Design review of the part built by this model. Coordinates are the model's own, in mm. A direction names the side the tool comes from. Round coordinates to 2 decimals unless told otherwise and drop trailing zeros. Order: outer loops, then holes, each group sorted by start corner. A loop starts at its lowest first (then second) coordinate and runs counter-clockwise, first axis right, second up. Notation, with made-up numbers: M 34,9 L 90,9 A22 ccw 90,45 Z; hole C 36,-20 d3. An arc over 180 degrees is marked long. Use a Markdown table: item, result. Add a question column.
(1) The part is to be moulded in two halves that separate along X. For faces 4 (the face through (-46, 5, 0)), 5 (the face through (-44.8, 2, 20)), 6 (the face through (21.04, 1.04, 16.09)), 7 (the face through (-26.863, 1.035, 35.391)), say which applies: released by +X, released by -X, zero draft, split by the parting line, or undercut.
(2) Take a section at A-A (x = 0). Write out the cut boundary in (y, z), then the cut area to 3 significant figures.
(3) Take a section at B-B (z = 0). Write out the cut boundary in (x, y), then the cut area to 3 significant figures.
(4) Take a section at D-D (x = -18). Write out the cut boundary in (y, z), then the cut area to 3 significant figures.
(5) To check wall thickness, follow probe 1 along Z at (x, y) = (0, 1.75); probe 2 along X at (y, z) = (1.3, -23). State the ranges of each line that lie inside material, in increasing order. Write a range as from..to.
(6) For pin 1 (1.5 mm diameter, centred on x = 19, z = 45.5, fed in from -Y); pin 2 (1.5 mm diameter, centred on x = 47, y = 3.5, fed in from +Z); pin 3 (1.1 mm diameter, centred on y = 2.5, z = -21.5, fed in from -X); pin 4 (2.5 mm diameter, centred on y = 2.5, z = -46.5, fed in from +X), all flat-tipped, find the tip position at first contact; note any pin that passes through.
(7) Machinability: for faces 1 (the face through (46, 1.2, 20)), 2 (the face through (10, 2.1, -10)), 3 (the face through (9.8, 1, -4.1)), which of the approach directions +Z, -Z, +X, -X, +Y, -Y give a long, thin tool a straight path to every point of the face, cutting with its end or side? Answer none if there is none.
(8) Take a section at C-C (z = -33). Write out the cut boundary in (x, y).
```python
from build123d import *

# Parameters (mm, degrees)
SKETCH1_R           = 5
BOSS_EXTRUDE1_DEPTH = 2.1
BOSS_EXTRUDE2_DEPTH = 2.9
SKETCH3_W           = 10.2
SKETCH3_H           = 3.8
CUT_EXTRUDE1_DEPTH  = 3
CIRPATTERN1_COUNT   = 4
CHAMFER1_SIZE       = 1


with BuildPart() as part:
    # Sketch1 → Boss-Extrude1 (new body)
    with BuildSketch(Plane(origin=(0, 0, 0), x_dir=(1, 0, 0), z_dir=(0, 1, 0))):
        Polygon((-47.8, -41.4), (-47.8, 41.4), (-41.4, 41.4), (-41.4, 47.8), (41.4, 47.8), (41.4, 41.4), (47.8, 41.4), (47.8, -41.4), (41.4, -41.4), (41.4, -47.8), (-41.4, -47.8), (-41.4, -41.4), align=None)
        Circle(SKETCH1_R, mode=Mode.SUBTRACT)
        with BuildLine():
            Line((-30.971572875, -26.021825407), (-10.834000483, -5.884253014))
            ThreePointArc((-10.834000483, -5.884253014), (-9.821178524, -4.171534398), (-9.758876863, -2.182732778))
            ThreePointArc((-9.758876863, -2.182732778), (-10, 0), (-9.758876863, 2.182732778))
            ThreePointArc((-9.758876863, 2.182732778), (-9.821178524, 4.171534398), (-10.834000483, 5.884253014))
            Line((-10.834000483, 5.884253014), (-30.971572875, 26.021825407))
            ThreePointArc((-30.971572875, 26.021825407), (-35.330733729, 26.888916412), (-37.8, 23.193398282))
            Line((-37.8, 23.193398282), (-37.8, -23.193398282))
            ThreePointArc((-37.8, -23.193398282), (-35.330733729, -26.888916412), (-30.971572875, -26.021825407))
        make_face(mode=Mode.SUBTRACT)
        with BuildLine():
            Line((-26.021825407, -30.971572875), (-5.884253014, -10.834000483))
            ThreePointArc((-5.884253014, -10.834000483), (-4.171534398, -9.821178524), (-2.182732778, -9.758876863))
            ThreePointArc((-2.182732778, -9.758876863), (0, -10), (2.182732778, -9.758876863))
            ThreePointArc((2.182732778, -9.758876863), (4.171534398, -9.821178524), (5.884253014, -10.834000483))
            Line((5.884253014, -10.834000483), (26.021825407, -30.971572875))
            ThreePointArc((26.021825407, -30.971572875), (26.888916412, -35.330733729), (23.193398282, -37.8))
            Line((23.193398282, -37.8), (-23.193398282, -37.8))
            ThreePointArc((-23.193398282, -37.8), (-26.888916412, -35.330733729), (-26.021825407, -30.971572875))
        make_face(mode=Mode.SUBTRACT)
        with BuildLine():
            Line((30.971572875, -26.021825407), (10.834000483, -5.884253014))
            ThreePointArc((10.834000483, -5.884253014), (9.821178524, -4.171534398), (9.758876863, -2.182732778))
            ThreePointArc((9.758876863, -2.182732778), (10, 0), (9.758876863, 2.182732778))
            ThreePointArc((9.758876863, 2.182732778), (9.821178524, 4.171534398), (10.834000483, 5.884253014))
            Line((10.834000483, 5.884253014), (30.971572875, 26.021825407))
            ThreePointArc((30.971572875, 26.021825407), (35.330733729, 26.888916412), (37.8, 23.193398282))
            Line((37.8, 23.193398282), (37.8, -23.193398282))
            ThreePointArc((37.8, -23.193398282), (35.330733729, -26.888916412), (30.971572875, -26.021825407))
        make_face(mode=Mode.SUBTRACT)
        with BuildLine():
            Line((-26.021825407, 30.971572875), (-5.884253014, 10.834000483))
            ThreePointArc((-5.884253014, 10.834000483), (-4.171534398, 9.821178524), (-2.182732778, 9.758876863))
            ThreePointArc((-2.182732778, 9.758876863), (0, 10), (2.182732778, 9.758876863))
            ThreePointArc((2.182732778, 9.758876863), (4.171534398, 9.821178524), (5.884253014, 10.834000483))
            Line((5.884253014, 10.834000483), (26.021825407, 30.971572875))
            ThreePointArc((26.021825407, 30.971572875), (26.888916412, 35.330733729), (23.193398282, 37.8))
            Line((23.193398282, 37.8), (-23.193398282, 37.8))
            ThreePointArc((-23.193398282, 37.8), (-26.888916412, 35.330733729), (-26.021825407, 30.971572875))
        make_face(mode=Mode.SUBTRACT)
    extrude(amount=BOSS_EXTRUDE1_DEPTH)

    # Sketch2 → Boss-Extrude2 (add)
    with BuildSketch(Plane(origin=(0, 2.1, 0), x_dir=(1, 0, 0), z_dir=(0, 1, 0))):
        Polygon((-47.8, -41.4), (-41.4, -41.4), (-41.4, -47.8), (41.4, -47.8), (41.4, -41.4), (47.8, -41.4), (47.8, 41.4), (41.4, 41.4), (41.4, 47.8), (-41.4, 47.8), (-41.4, 41.4), (-47.8, 41.4), align=None)
        Polygon((-42.8, 34.314718626), (-42.8, -34.314718626), (-34.314718626, -42.8), (34.314718626, -42.8), (42.8, -34.314718626), (42.8, 34.314718626), (34.314718626, 42.8), (-34.314718626, 42.8), align=None, mode=Mode.SUBTRACT)
    extrude(amount=BOSS_EXTRUDE2_DEPTH)

    # Sketch3 → Cut-Extrude1 (cut)
    with BuildSketch(Plane.ZY.offset(47.8)):
        with Locations((20, 1.9)):
            Rectangle(SKETCH3_W, SKETCH3_H)
        with Locations((-20, 3.1)):
            Rectangle(SKETCH3_W, SKETCH3_H)
    cut_extrude1 = extrude(amount=-CUT_EXTRUDE1_DEPTH, mode=Mode.SUBTRACT)

    # CirPattern1: Cut-Extrude1 ×4 about axis
    cirpattern1_axis = Axis((0, 0, 0), (0, 1, 0))
    for i in range(1, CIRPATTERN1_COUNT):
        add(cut_extrude1.rotate(cirpattern1_axis, i * 360 / CIRPATTERN1_COUNT), mode=Mode.SUBTRACT)

    # Chamfer1
    chamfer1_edges = [part.edges().sort_by_distance(p)[0] for p in [
        (-38.557359313, 5, -38.557359313),
        (-42.8, 5, 0),
        (-38.557359313, 5, 38.557359313),
        (0, 5, 42.8),
        (38.557359313, 5, 38.557359313),
        (42.8, 5, 0),
        (38.557359313, 5, -38.557359313),
        (0, 5, -42.8),
    ]]
    chamfer(chamfer1_edges, length=CHAMFER1_SIZE)


solid = part.part
```
Verdict:
| question | item | result |
|---|---|---|
| 1 | face 4 | zero draft |
| 1 | face 5 | released by -X |
| 1 | face 6 | undercut |
| 1 | face 7 | undercut |
| 2 | outline | M 0,-47.8 L 5,-47.8 L 5,-43.8 L 4,-42.8 L 2.1,-42.8 L 2.1,-37.8 L 0,-37.8 Z; M 0,-10 L 2.1,-10 L 2.1,-5 L 0,-5 Z; M 0,5 L 2.1,5 L 2.1,10 L 0,10 Z; M 0,37.8 L 2.1,37.8 L 2.1,42.8 L 4,42.8 L 5,43.8 L 5,47.8 L 0,47.8 Z |
| 2 | area | 91.0 mm^2 |
| 3 | outline | M -47.8,0 L -37.8,0 L -37.8,2.1 L -42.8,2.1 L -42.8,4 L -43.8,5 L -47.8,5 Z; M -10,0 L -5,0 L -5,2.1 L -10,2.1 Z; M 5,0 L 10,0 L 10,2.1 L 5,2.1 Z; M 37.8,0 L 47.8,0 L 47.8,5 L 43.8,5 L 42.8,4 L 42.8,2.1 L 37.8,2.1 Z |
| 3 | area | 91.0 mm^2 |
| 4 | outline | M 0,-44.8 L 3.8,-44.8 L 3.8,-47.8 L 5,-47.8 L 5,-43.8 L 4,-42.8 L 2.1,-42.8 L 2.1,-37.8 L 0,-37.8 Z; M 0,-22.95 L 2.1,-22.95 L 2.1,-13.05 L 0,-13.05 Z; M 0,13.05 L 2.1,13.05 L 2.1,22.95 L 0,22.95 Z; M 0,37.8 L 2.1,37.8 L 2.1,42.8 L 4,42.8 L 5,43.8 L 5,44.8 L 1.2,44.8 L 1.2,47.8 L 0,47.8 Z |
| 4 | area | 88.8 mm^2 |
| 5 | probe 1 | z = -47.8..-37.8, -10..-5, 5..10, 37.8..47.8 |
| 5 | probe 2 | x = -44.8..-37.8, -27.95..-18.05, 18.05..27.95, 37.8..44.8 |
| 6 | pin 1 | stops at y = 0 |
| 6 | pin 2 | stops at z = 41.4 |
| 6 | pin 3 | stops at x = -44.8 |
| 6 | pin 4 | stops at x = 41.4 |
| 7 | face 1 | +X, +Y |
| 7 | face 2 | +Y |
| 7 | face 3 | +Y, -Y |
| 8 | outline | M -47.8,0 L -27.11,0 L -27.11,2.1 L -42.8,2.1 L -42.8,4 L -43.8,5 L -47.8,5 Z; M 27.11,0 L 47.8,0 L 47.8,5 L 43.8,5 L 42.8,4 L 42.8,2.1 L 27.11,2.1 Z |
